Verification items for the finished model (mm, model axes). A direction names the side the tool comes from. Give positions to 0.01 mm unless a question says otherwise; leave off trailing zeros. Order: outer loops, then holes, each group sorted by start corner. A loop starts at its lowest first (then second) coordinate and runs counter-clockwise, first axis right, second up. Notation, with made-up numbers: (50, 28.5) - (108, 28.5) arc R8 ccw to (108, 34.5) - close; hole circle Ø4 at (42, 20.25). An arc over 180 degrees is marked (long way). Answer as a JSON object with one key per item and string values.
```python
from build123d import *

# Parameters (mm, degrees)
F1_DEPTH  = 12.7
F0_W      = 163.3856055679
F0_H      = 27.0547205253
F0_H_2    = 34.7771560773
F0_H_3    = 32.1148465989
F2_DEPTH  = 12.192
F0_W_2    = 6.2235964999
F0_H_4    = 43.18
F0_W_3    = 3.7542508378
F0_W_4    = 9.6248776398
F0_W_5    = 7.4676067315
F7_R      = 32.7809954098
F7_R_2    = 6.2235964999
F8_DEPTH  = 6.35
F9_R      = 34.1304188129
F9_R_2    = 9.6248776398
F10_DEPTH = 6.35
F11_R     = 31.6050614304
F11_R_2   = 7.4676067315
F12_DEPTH = 6.35
F13_R     = 28.7772808224
F13_R_2   = 3.7542508378
F14_DEPTH = 6.35


with BuildPart() as f1:
    # F0 (on Front) → F1 (new body, symmetric)
    with BuildSketch(Plane.XZ):
        with BuildLine():
            Line((186.7009509993, 49.238986743), (161.7247212493, 82.55))
            Line((161.7247212493, 82.55), (-161.7247212493, 82.55))
            Line((-161.7247212493, 82.55), (-178.912508309, 44.6288234264))
            Line((-178.912508309, 44.6288234264), (-196.4037567377, 44.6288234264))
            Line((-196.4037567377, 44.6288234264), (-202.6273532376, 44.6288234264))
            Line((-202.6273532376, 44.6288234264), (-218.5374638219, 44.6288234264))
            Line((-218.5374638219, 44.6288234264), (-218.5374638219, 77.9398366834))
            ThreePointArc((-218.5374638219, 77.9398366834), (-271.8769801908, 0.258229293), (-222.4398309941, -79.9633663813))
            Line((-222.4398309941, -79.9633663813), (-222.4398309941, -46.6523531243))
            Line((-222.4398309941, -46.6523531243), (-206.3816040754, -46.6523531243))
            Line((-206.3816040754, -46.6523531243), (-202.6273532376, -46.6523531243))
            Line((-202.6273532376, -46.6523531243), (-182.8148754811, -46.6523531243))
            Line((-182.8148754811, -46.6523531243), (-161.7247212493, -82.55))
            Line((-161.7247212493, -82.55), (161.7247212493, -82.55))
            Line((161.7247212493, -82.55), (186.7009509993, -49.238986743))
            Line((186.7009509993, -49.238986743), (199.0458220243, -49.238986743))
            Line((199.0458220243, -49.238986743), (206.5134287558, -49.238986743))
            Line((206.5134287558, -49.238986743), (226.3259065123, -49.238986743))
            Line((226.3259065123, -49.238986743), (226.3259065123, -82.55))
            ThreePointArc((226.3259065123, -82.55), (287.2935352333, 0), (226.3259065123, 82.55))
            Line((226.3259065123, 82.55), (226.3259065123, 49.238986743))
            Line((226.3259065123, 49.238986743), (206.5134287558, 49.238986743))
            Line((206.5134287558, 49.238986743), (196.888551116, 49.238986743))
            Line((196.888551116, 49.238986743), (186.7009509993, 49.238986743))
        make_face()
        Polygon((137.5162151193, -14.8585150018), (137.5162151193, -46.9733616008), (-25.8693904485, -46.9733616008), (-25.8693904485, -14.8585150018), (-25.8693904485, 19.9186410755), (-25.8693904485, 46.9733616008), (137.5162151193, 46.9733616008), (137.5162151193, 19.9186410755), align=None, mode=Mode.SUBTRACT)
    extrude(amount=F1_DEPTH, both=True)

    # F0 (on Front) → F2 (join)
    with BuildSketch(Plane.XZ):
        with Locations((55.8234123354, 33.4460013381)):
            Rectangle(F0_W, F0_H)
        with Locations((55.8234123354, 2.5300630368)):
            Rectangle(F0_W, F0_H_2)
        with Locations((55.8234123354, -30.9159383013)):
            Rectangle(F0_W, F0_H_3)
    extrude(amount=-F2_DEPTH)

    # F0 (on Front) → F3 (revolve)
    with BuildSketch(Plane.XZ):
        with Locations((-199.5155549877, 66.2188234264)):
            Rectangle(F0_W_2, F0_H_4)
    revolve(axis=Axis((-196.4037567377, 0, 66.2188234264), (0, 0, 1)))

    # F0 (on Front) → F4 (revolve)
    with BuildSketch(Plane.XZ):
        with Locations((-204.5044786565, -68.2423531243)):
            Rectangle(F0_W_3, F0_H_4)
    revolve(axis=Axis((-202.6273532376, 0, -68.2423531243), (0, 0, -1)))

    # F0 (on Front) → F5 (revolve)
    with BuildSketch(Plane.XZ):
        with Locations((201.7009899359, 70.828986743)):
            Rectangle(F0_W_4, F0_H_4)
    revolve(axis=Axis((206.5134287558, 0, 70.828986743), (0, 0, 1)))

    # F0 (on Front) → F6 (revolve)
    with BuildSketch(Plane.XZ):
        with Locations((202.7796253901, -70.828986743)):
            Rectangle(F0_W_5, F0_H_4)
    revolve(axis=Axis((206.5134287558, 0, -70.828986743), (0, 0, -1)))

    # F7 (on face) → F8 (join, symmetric)
    with BuildSketch(Plane.XY.offset(87.8088234264)):
        with Locations((-196.4037567377, 0)):
            Circle(F7_R)
        with Locations((-196.4037567377, 0)):
            Circle(F7_R_2, mode=Mode.SUBTRACT)
    extrude(amount=F8_DEPTH, both=True)

    # F9 (on face) → F10 (join, symmetric)
    with BuildSketch(Plane.XY.offset(92.418986743)):
        with Locations((206.5134287558, 0)):
            Circle(F9_R)
        with Locations((206.5134287558, 0)):
            Circle(F9_R_2, mode=Mode.SUBTRACT)
    extrude(amount=F10_DEPTH, both=True)

    # F11 (on face) → F12 (join, symmetric)
    with BuildSketch(Plane(origin=(0, 0, -92.418986743), x_dir=(1, 0, 0), z_dir=(0, 0, -1))):
        with Locations((206.5134287558, 0)):
            Circle(F11_R)
        with Locations((206.5134287558, 0)):
            Circle(F11_R_2, mode=Mode.SUBTRACT)
    extrude(amount=F12_DEPTH, both=True)

    # F13 (on face) → F14 (join, symmetric)
    with BuildSketch(Plane(origin=(0, 0, -89.8323531243), x_dir=(1, 0, 0), z_dir=(0, 0, -1))):
        with Locations((-202.6273532376, 0)):
            Circle(F13_R)
        with Locations((-202.6273532376, 0)):
            Circle(F13_R_2, mode=Mode.SUBTRACT)
    extrude(amount=F14_DEPTH, both=True)


solid = f1.part
```
(1) Material ranges on line 1 along Z through (x, y) = (187.5, -4.5); line 2 along X through (y, z) = (0, -93); line 3 along Z through (x, y) = (-17, -11), recorded low to high. Write a range as [from, to].
Computed values:
{"line 1": "z = [-98.77, -86.07], [-49.24, 49.24], [86.07, 98.77]", "line 2": "x = [-231.4, -206.38], [-198.87, -173.85], [174.91, 199.05], [213.98, 238.12]", "line 3": "z = [-82.55, -46.97], [46.97, 82.55]"}
(2) Release check for a two-part mould opening along Z. For faces 1 (the flat face through (-25.869, -6, -1)), 2 (the cylindrical face through (239.07, 10.25, 92.51)), 3 (the flat face through (207, 0, -92.419)), 4 (the flat face through (-197, -7, 94.159)) record: pulls with the +Z half, pulls with the -Z half, needs draft (parallel to the pull), parting line crosses it, or undercut.
Computed values:
{"face 1": "undercut", "face 2": "needs draft", "face 3": "pulls with the -Z half", "face 4": "pulls with the +Z half"}
(3) Section check C-C (x = -58). Record the cut outline in (y, z).
Computed values:
{"outline": "(-12.7, -82.55) - (12.7, -82.55) - (12.7, 82.55) - (-12.7, 82.55) - close"}
(4) Section check B-B (z = -16.5). Record the cut outline in (x, y), then the cut area to 3 significant figures.
Computed values:
{"outline": "(-270.66, -12.7) - (-25.87, -12.7) - (-25.87, 0) - (137.52, 0) - (137.52, -12.7) - (285.7, -12.7) - (285.7, 12.7) - (137.52, 12.7) - (137.52, 12.19) - (-25.87, 12.19) - (-25.87, 12.7) - (-270.66, 12.7) - close", "area": "12,000 mm²"}
(5) Access from +Z, -Z, +X, -X, +Y, -Y to the whole of each face (thin tool, end or side, straight path). Record for faces 5 (the cylindrical face through (-190.655, -2.384, 90.939)), 6 (the flat face through (214, -7, 98.769)), 7 (the flat face through (174.39, -0.18, 65.66)), 8 (the flat face through (-2, 0, -82.55)), 9 (the flat face through (213, 7, -86.069)).
Computed values:
{"face 5": "+Z", "face 6": "+Z, +X, -X, +Y, -Y", "face 7": "+Y, -Y", "face 8": "-Z, +Y, -Y", "face 9": "none"}
(6) Gauge pin test, flat ends, axial feed: pin 1 Ø12 at (x, y) = (207.5, -1) entering from -Z; pin 2 Ø6 at (x, y) = (-199, 3) entering from +Z; pin 3 Ø2 at (y, z) = (-14.5, -17) entering from -X; pin 4 Ø10 at (x, y) = (89.5, -6) entering from +Z. Record the tip position at first contact, or that the pin passes through.
Computed values:
{"pin 1": "stops at z = -92.42", "pin 2": "stops at z = 94.16", "pin 3": "passes through", "pin 4": "stops at z = 82.55"}
(7) Section check A-A (x = 19). Record the cut outline in (y, z), then the cut area to 3 significant figures.
Computed values:
{"outline": "(-12.7, -82.55) - (12.7, -82.55) - (12.7, -46.97) - (12.19, -46.97) - (12.19, 46.97) - (12.7, 46.97) - (12.7, 82.55) - (-12.7, 82.55) - (-12.7, 46.97) - (0, 46.97) - (0, -46.97) - (-12.7, -46.97) - close", "area": "2,950 mm²"}
